Answer from the drawing. Dimensions are ordinates in mm from the lowest x, y and z of the part. Coordinates: 2 decimals unless noted, no trailing zeros. Order: outer loops, then holes, each group sorted by start corner. A loop starts at its lowest first (then second) coordinate and runs counter-clockwise, first axis right, second up. Notation, with made-up numbers: (11, -4.5) - (29, -4.5) arc R22 cw to (29, 4.5) - close; hole circle Ø4 at (22.25, -10). An arc over 180 degrees is marked (long way). Answer as a JSON object with one key per item and string values. Group by question number.
1) Section A-A (z = 300) is taken. Give the vertices of the cut face in (x, y).
2) Section C-C (x = 92) is taken. Give the vertices of the cut face in (y, z), plus the area to 3 significant figures.
3) Section D-D (y = 139) is taken. Give the vertices of the cut face in (x, z).
4) The mould has two halves that part along Y. Classify the marked faces 1, 2 and 3: released by +Y, released by -Y, zero draft, split by the parting line, or undercut.
5) Each of these flat-tipped pins is pushed along its axis until it touches: P1, Ø6, axis at x = 50, z = 381, coming from the +Y side; P2, Ø1.5, axis at x = 44.5, y = 391.5, coming from the +Z side (3 decimals); P3, Ø6, axis at x = 78, y = 108, coming from the +Z side; P4, Ø8, axis at y = 469, z = 372.5, coming from the -X side. Where does it stop, or does it pass through?
6) Find the intervals of material crossed by line 1 along Y through (x, z) = (67.5, 300); line 2 along Y through (x, z) = (79, 300); line 3 along Z through (x, y) = (66.5, 94), in increasing order.
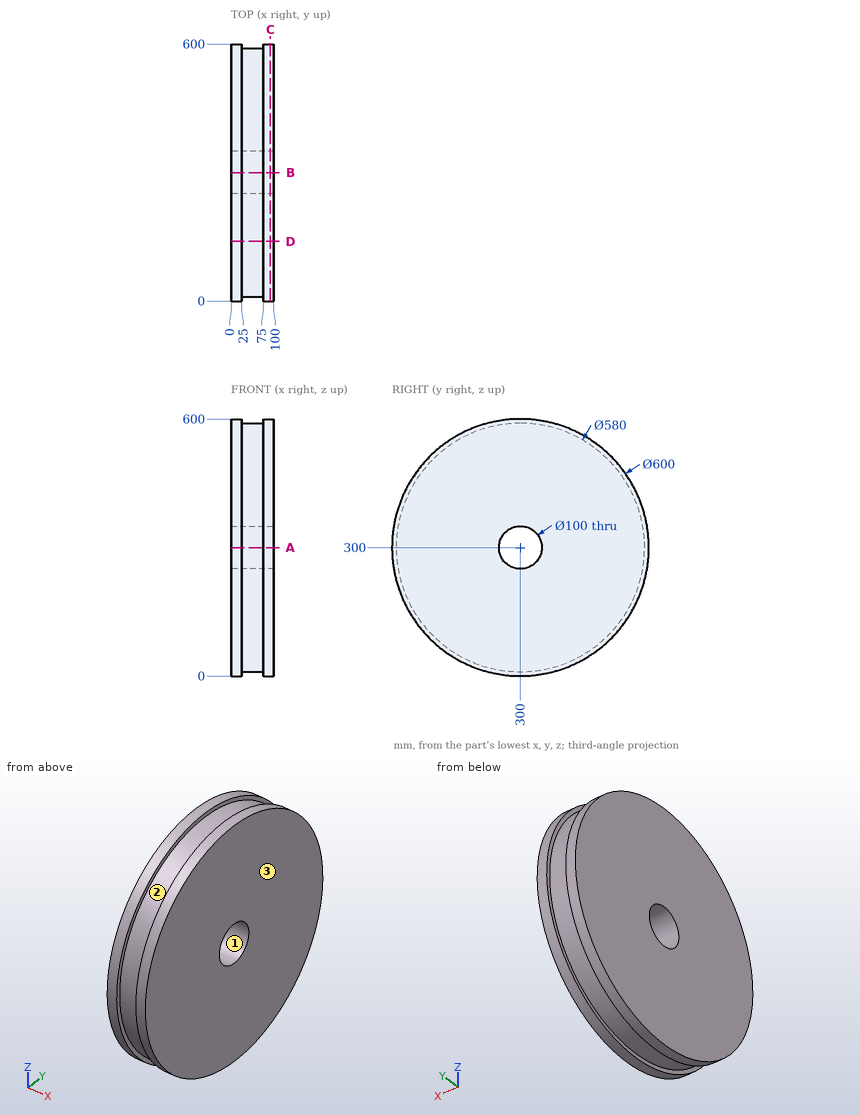
Report:
{
 "1": {"outline": "(0, 0) - (25, 0) - (25, 10) - (75, 10) - (75, 0) - (100, 0) - (100, 250) - (0, 250) - close; (0, 350) - (100, 350) - (100, 600) - (75, 600) - (75, 590) - (25, 590) - (25, 600) - (0, 600) - close"},
 "2": {"outline": "circle Ø600 at (300, 300); hole circle Ø100 at (300, 300)", "area": "275,000 mm²"},
 "3": {"outline": "(0, 46.86) - (25, 46.86) - (25, 58.8) - (75, 58.8) - (75, 46.86) - (100, 46.86) - (100, 553.14) - (75, 553.14) - (75, 541.2) - (25, 541.2) - (25, 553.14) - (0, 553.14) - close"},
 "4": {"face 1": "undercut", "face 2": "split by the parting line", "face 3": "zero draft"},
 "5": {"P1": "stops at y = 579.31", "P2": "stops at z = 575.435", "P3": "stops at z = 532.98", "P4": "stops at x = 0"},
 "6": {"line 1": "y = 10 to 250, 350 to 590", "line 2": "y = 0 to 250, 350 to 600", "line 3": "z = 95.88 to 504.12"}
}
